For this review, take the finished solid that the model builds, in its own axes (mm). A direction names the side the tool comes from. Coordinates: 2 decimals unless noted, no trailing zeros. Loops run counter-clockwise (first coordinate to the right, second up) from the corner with the lowest first, then second, coordinate; pieces in that order, holes last. Notation, with made-up numbers: (84.5, -7) - (115.5, -7) arc R6 cw to (115.5, -3) - close; hole circle Ø7 at (29.25, 36.5). An arc over 180 degrees is marked (long way). Use one line per item in the form item = value. Start each with the question number.
1. Add section C-C on y = -66. Give the boundary of the cut face in (x, z) (3 decimals).
2. To check wall thickness, follow probe 1 along X at (y, z) = (-48.5, 1.35); probe 2 along X at (y, z) = (48, 3); probe 3 along X at (y, z) = (-45, 2.35). State the ranges of each line that lie inside material, in increasing order.
3. Machinability: for faces 4 (the face through (63.825, -9.89, 1.565)), 5 (the face through (-59.09, 26.07, 1.57)), 6 (the face through (-32.04, -55.69, 1.57)), 7 (the face through (9.89, 63.825, 1.565)), which of the approach directions +Z, -Z, +X, -X, +Y, -Y give a long, thin tool a straight path to every point of the face, cutting with its end or side? Answer none if there is none.
4. For pin 1 Ø1 at (y, z) = (50.5, 0.5) entering from -X, flat-tipped, find the tip position at first contact; note if it passes through.
5. Add section D-D on y = -20. Give the boundary of the cut face in (x, z) (3 decimals), and give its area (3 significant figures).
6. Add section A-A on x = 0. Give the boundary of the cut face in (y, z) (3 decimals).
7. Draft analysis for pull direction Y (two halves, no side actions). For faces 1 (the face through (16, 1, 3.175)), 2 (the face through (45.5, -45.36, 1.57)), 3 (the face through (0.1, -64.25, 1.57)), state which applies: +Y half, -Y half, draft (parallel to the pull), parting line (faces both ways), or undercut.
```python
from build123d import *

# Parameters (mm, degrees)
F0_R     = 9.525
F1_DEPTH = 3.175


with BuildPart() as f1:
    # F0 (on Top) → F1 (new body)
    with BuildSketch(Plane.XY):
        Polygon((34.528738, 68.326658), (17.376506, 49.592707), (15.66796, 74.935178), (3.948879, 52.400247), (-4.260564, 76.436991), (-9.747858, 51.636797), (-23.898738, 72.729748), (-22.780294, 47.354384), (-41.908252, 64.066093), (-34.260291, 39.844849), (-57.061788, 51.03644), (-43.405506, 29.619953), (-68.326658, 34.528738), (-49.592707, 17.376506), (-74.935178, 15.66796), (-52.400247, 3.948879), (-76.436991, -4.260564), (-51.636797, -9.747858), (-72.729748, -23.898738), (-47.354384, -22.780294), (-64.066093, -41.908252), (-39.844849, -34.260291), (-51.03644, -57.061788), (-29.619953, -43.405506), (-34.528738, -68.326658), (-17.376506, -49.592707), (-15.66796, -74.935178), (-3.948879, -52.400247), (4.260564, -76.436991), (9.747858, -51.636797), (23.898738, -72.729748), (22.780294, -47.354384), (41.908252, -64.066093), (34.260291, -39.844849), (57.061788, -51.03644), (43.405506, -29.619953), (68.326658, -34.528738), (49.592707, -17.376506), (74.935178, -15.66796), (52.400247, -3.948879), (76.436991, 4.260564), (51.636797, 9.747858), (72.729748, 23.898738), (47.354384, 22.780294), (64.066093, 41.908252), (39.844849, 34.260291), (51.03644, 57.061788), (29.619953, 43.405506), align=None)
        Circle(F0_R, mode=Mode.SUBTRACT)
    extrude(amount=F1_DEPTH)


solid = f1.part
```
Conclusion:
q1.outline = (-34.07, 0) - (-32.399, 0) - (-32.399, 3.175) - (-34.07, 3.175) - close; (-16.27, 0) - (-11.021, 0) - (-11.021, 3.175) - (-16.27, 3.175) - close; (0.696, 0) - (6.57, 0) - (6.57, 3.175) - (0.696, 3.175) - close; (19.384, 0) - (23.602, 0) - (23.602, 3.175) - (19.384, 3.175) - close
q2.probe_1 = -46.83 to -37.61, -30.62 to 22.83, 24.09 to 36.99, 51.89 to 55.44
q2.probe_2 = -55.13 to -50.88, -36.84 to -23.52, -22.81 to 30.52, 36.83 to 46.59
q2.probe_3 = -45.12 to -32.12, -29.93 to 35.89, 44.76 to 53.21
q3.face_4 = +Z, -Z, +X
q3.face_5 = +Z, -Z, -X
q3.face_6 = +Z, -Z
q3.face_7 = +Z, -Z, +Y
q4.pin_1 = -57.04
q5.outline = (-66.918, 0) - (52.458, 0) - (52.458, 3.175) - (-66.918, 3.175) - close
q5.area = 379 mm^2
q6.outline = (-63.962, 0) - (-9.525, 0) - (-9.525, 3.175) - (-63.962, 3.175) - close; (9.525, 0) - (63.962, 0) - (63.962, 3.175) - (9.525, 3.175) - close
q7.face_1 = draft
q7.face_2 = undercut
q7.face_3 = -Y half
